Design review of the part built by this model. Coordinates are the model's own, in mm. Face numbers are marked on the shaded views. A direction names the side the tool comes from. Round coordinates to 2 decimals unless told otherwise and drop trailing zeros. Order: outer loops, then holes, each group sorted by start corner. A loop starts at its lowest first (then second) coordinate and runs counter-clockwise, first axis right, second up. Notation, with made-up numbers: (1, 31.5) - (27, 31.5) arc R12 cw to (27, 48.5) - close; hole circle Ø11 at (-23, 56.5). An arc over 180 degrees is marked (long way). Answer as a JSON object with one key per item and string values. Group by question number.
from build123d import *

# Parameters (mm, degrees)
BOSS_EXTRUDE1_DEPTH      = 6
FILLET1_R                = 1.5
BOSS_EXTRUDE2_DEPTH      = 25
BOSS_EXTRUDE2_DEPTH_BACK = 25
CUT_EXTRUDE1_DEPTH       = 87.306907839
BOSS_EXTRUDE3_DEPTH      = 2
F_4_0_4_DIAMETER_HOLE1_D = 4
SKETCH15_R               = 3.75
CUT_EXTRUDE2_DEPTH       = 3
SKETCH16_W               = 5
SKETCH16_H               = 53
BOSS_EXTRUDE4_DEPTH      = 10
CUT_EXTRUDE3_DEPTH       = 87.525968801
CUT_EXTRUDE3_DEPTH_BACK  = 10


with BuildPart() as part:
    # Sketch1 → Boss-Extrude1 (new body)
    with BuildSketch(Plane(origin=(0, 0, 0), x_dir=(0, 0, -1), z_dir=(1, 0, 0))):
        Polygon((-9.55, 0), (9.55, 0), (7.017409876, -7.588543158), (0, -9.6), (-7.017409876, -7.588543158), align=None)
    extrude(amount=BOSS_EXTRUDE1_DEPTH)

    # Fillet1
    fillet1_edges = [part.edges().sort_by_distance(p)[0] for p in [
        (3, -7.588543158, -7.017409876),
        (3, -9.6, 0),
        (3, -7.588543158, 7.017409876),
    ]]
    fillet(fillet1_edges, radius=FILLET1_R)

    # Sketch2 → Boss-Extrude2 (add, two sides: drawn at the far end of the back side and taken through both)
    with BuildSketch(Plane.XY.offset(-BOSS_EXTRUDE2_DEPTH_BACK)):
        Polygon((0, 0), (-19.052558883, 11), (-50.683324779, -43.786093614), (-42.023070741, -48.786093614), (-14.523070741, -1.154696406), (0, -9.539595208), align=None)
    extrude(amount=BOSS_EXTRUDE2_DEPTH + BOSS_EXTRUDE2_DEPTH_BACK)

    # Sketch10 → Cut-Extrude1 (cut, through all)
    with BuildSketch(Plane.XY.offset(25)):
        Polygon((6, 0), (6, -6.839154339), (5, 0), align=None)
    extrude(amount=-CUT_EXTRUDE1_DEPTH, mode=Mode.SUBTRACT)

    # Sketch14 → Boss-Extrude3 (add)
    with BuildSketch(Plane(origin=(-4.130765896, -7.154696406, 0), x_dir=(0.8660254037844397, -0.4999999999999982, 0), z_dir=(-0.4999999999999983, -0.8660254037844398, 0))):
        Polygon((-12, 25), (-12, -25), (4.769797604, -25), (4.769797604, 0), (4.769797604, 25), align=None)
    extrude(amount=BOSS_EXTRUDE3_DEPTH)

    # Ø4.0 (4) Diameter Hole1 (through all)
    with Locations(Plane(origin=(-19.052558883, 11, 0), x_dir=(0, 0, 1), z_dir=(-0.8660254037844399, 0.4999999999999977, 0))):
        with Locations((0, -40.261531792), (0, -55.261531792)):
            Hole(F_4_0_4_DIAMETER_HOLE1_D / 2)

    # Sketch15 → Cut-Extrude2 (cut)
    with BuildSketch(Plane(origin=(-19.052558883, 11, 0), x_dir=(-0.4999999999999977, -0.8660254037844399, 0), z_dir=(-0.8660254037844399, 0.4999999999999977, 0))):
        with Locations((40.261531792, 0)):
            Circle(SKETCH15_R)
        with Locations((55.261531792, 0)):
            Circle(SKETCH15_R)
    extrude(amount=-CUT_EXTRUDE2_DEPTH, mode=Mode.SUBTRACT)

    # Sketch16 → Boss-Extrude4 (add)
    with BuildSketch(Plane(origin=(-10.392304845, 6, 0), x_dir=(0, 0, -1), z_dir=(0.8660254037844398, -0.49999999999999795, 0))):
        with Locations((-22.5, -36.761531792)):
            Rectangle(SKETCH16_W, SKETCH16_H)
    boss_extrude4 = extrude(amount=BOSS_EXTRUDE4_DEPTH)

    # Mirror1: Boss-Extrude4 across plane
    add(boss_extrude4.mirror(Plane.XY))

    # Sketch17 → Cut-Extrude3 (cut, two sides: drawn at the far end of the back side and taken through both)
    with BuildSketch(Plane.XY.offset(-20).offset(-CUT_EXTRUDE3_DEPTH_BACK)):
        Polygon((-42.023070741, -48.786093614), (-6.862816703, -7.886747213), (-33.362816703, -53.786093614), align=None)
    extrude(amount=CUT_EXTRUDE3_DEPTH + CUT_EXTRUDE3_DEPTH_BACK, mode=Mode.SUBTRACT)


solid = part.part
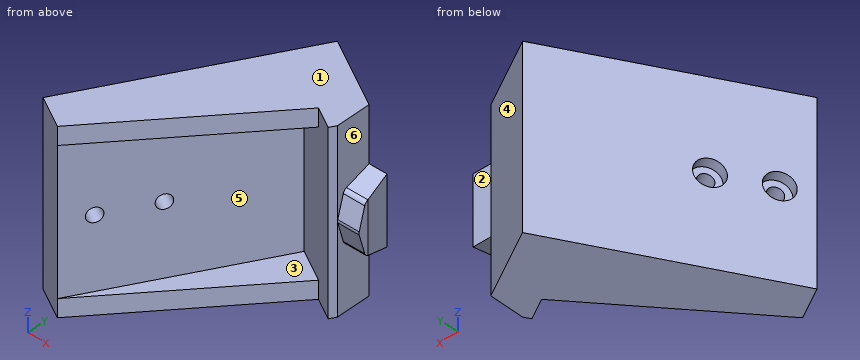
1. Take a section at D-D, the plane x = -35.5. Count the separate pieces of the cut face and the enclosed holes in it, then the cut area to 3 significant figures.
2. Take a section at C-C, the plane y = 6.5. Give the boundary of the cut face in (x, z), then the cut area to 3 significant figures.
3. Clearance check with flat-ended pins moving along their axes: P1, Ø1.5, axis at x = -23, y = -28.5, coming from the +Z side; P2, Ø1.5, axis at x = 3, z = -2.5, coming from the +Y side; P3, Ø1, axis at x = -39.5, z = 16, coming from the -Y side; P4, Ø1, axis at x = -22, z = 0.5, coming from the +Y side. State where each tip first meets the part, or that it passes through.
4. Take a section at B-B, the plane x = -8. Give the boundary of the cut face in (y, z), then the cut area to 3 significant figures.
5. To check wall thickness, follow line 1 (Z direction, x = -34.5, y = -40); line 2 (X direction, y = -43.5, z = 11.5); line 3 (X direction, y = -37, z = -9). State the ranges of each line that lie inside material, in increasing order. Write a range as from..to.
6. Tool access review of the marked faces 4, 5 and 6: name each direction out of +Z, -Z, +X, -X, +Y, -Y from which nothing blocks a thin tool from reaching the whole face with its end or side.
7. Mouldability with a two-part tool opening along Z and no side actions: class the marked faces 1, 2 and 3 as pulls with the +Z half, pulls with the -Z half, needs draft (parallel to the pull), parting line crosses it, or undercut.
8. Take a section at A-A, the plane z = 19. Give the boundary of the cut face in (x, y), then the cut area to 3 significant figures.
Response values:
{
 "1": {"separate pieces": "1", "enclosed holes": "2", "area": "1,010 mm2"},
 "2": {"outline": "(-21.65, -25) - (-11.26, -25) - (-11.26, 25) - (-21.65, 25) - close", "area": "520 mm2"},
 "3": {"P1": "through", "P2": "y = 0", "P3": "y = -45.28", "P4": "y = 6.76"},
 "4": {"outline": "(-9.21, -25) - (4.62, -25) - (4.62, 25) - (-9.21, 25) - (-9.21, 20) - (-7.23, 20) - (-7.23, -20) - (-9.21, -20) - close", "area": "612 mm2"},
 "5": {"line 1": "-25..-20, 20..25", "line 2": "-50.52..-38.97", "line 3": "-46.77..-35.22"},
 "6": {"face 4": "+Z, -Z, +X, +Y", "face 5": "-Y", "face 6": "+Z, +X, -Y"},
 "7": {"face 1": "pulls with the +Z half", "face 2": "needs draft", "face 3": "undercut"},
 "8": {"outline": "(-50.68, -43.79) - (-42.02, -48.79) - (-15.52, -2.89) - (-1, -11.27) - (0, -9.54) - (0, 0) - (-19.05, 11) - close", "area": "785 mm2"}
}
